```python
from build123d import *

# Parameters (mm, degrees)
SKETCH1_W           = 220
SKETCH1_H           = 30
BOSS_EXTRUDE1_DEPTH = 10
SKETCH2_W           = 23.523691572
SKETCH2_H           = 30
SKETCH2_R           = 11.1
BOSS_EXTRUDE3_DEPTH = 10
SKETCH6_R           = 1.5
CUT_EXTRUDE2_DEPTH  = 10
CUT_EXTRUDE3_START  = -10
SKETCH4_R           = 4
CUT_EXTRUDE3_DEPTH  = 4
SKETCH7_R           = 1.5
CUT_EXTRUDE4_DEPTH  = 14
CUT_EXTRUDE5_DEPTH  = 10
FILLET1_R           = 10


with BuildPart() as part:
    # Sketch1 → Boss-Extrude1 (new body)
    with BuildSketch(Plane(origin=(0, 0, 0), x_dir=(1, 0, 0), z_dir=(0, 1, 0))):
        Rectangle(SKETCH1_W, SKETCH1_H)
    extrude(amount=BOSS_EXTRUDE1_DEPTH)

    # Sketch2 → Boss-Extrude3 (add)
    with BuildSketch(Plane(origin=(0, 10, 0), x_dir=(1, 0, 0), z_dir=(0, 1, 0))):
        with Locations((-98.238154214, 0)):
            Rectangle(SKETCH2_W, SKETCH2_H)
        with Locations(Location((-98.238154214, 0, 0), (0, 0, 270))):
            Circle(SKETCH2_R, mode=Mode.SUBTRACT)
    extrude(amount=BOSS_EXTRUDE3_DEPTH)

    # Sketch6 → Cut-Extrude2 (cut)
    with BuildSketch(Plane.XY.offset(15)):
        with Locations((-98.238154214, 15)):
            Circle(SKETCH6_R)
    extrude(amount=-CUT_EXTRUDE2_DEPTH, mode=Mode.SUBTRACT)

    # Sketch4 → Cut-Extrude3 (cut)
    with BuildSketch(Plane(origin=(0, 10, 0), x_dir=(1, 0, 0), z_dir=(0, 1, 0)).offset(CUT_EXTRUDE3_START)):
        with Locations(Location((90, 0, 0), (0, 0, 90))):
            Circle(SKETCH4_R)
    extrude(amount=CUT_EXTRUDE3_DEPTH, mode=Mode.SUBTRACT)

    # Sketch7 → Cut-Extrude4 (cut)
    with BuildSketch(Plane(origin=(0, 4, 0), x_dir=(-1, 0, 0), z_dir=(0, -1, 0))):
        with Locations(Location((-90, 0, 0), (0, 0, 90))):
            Circle(SKETCH7_R)
    extrude(amount=-CUT_EXTRUDE4_DEPTH, mode=Mode.SUBTRACT)

    # Sketch8 → Cut-Extrude5 (cut)
    with BuildSketch(Plane(origin=(0, 10, 0), x_dir=(1, 0, 0), z_dir=(0, 1, 0))):
        Polygon((110, -15), (110, 0), (95, -15), align=None)
        Polygon((110, 15), (95, 15), (110, 0), align=None)
    extrude(amount=-CUT_EXTRUDE5_DEPTH, mode=Mode.SUBTRACT)

    # Fillet1
    fillet1_edges = [part.edges().sort_by_distance(p)[0] for p in [
        (110, 5, 0),
        (95, 5, 15),
        (95, 5, -15),
    ]]
    fillet(fillet1_edges, radius=FILLET1_R)


solid = part.part
```
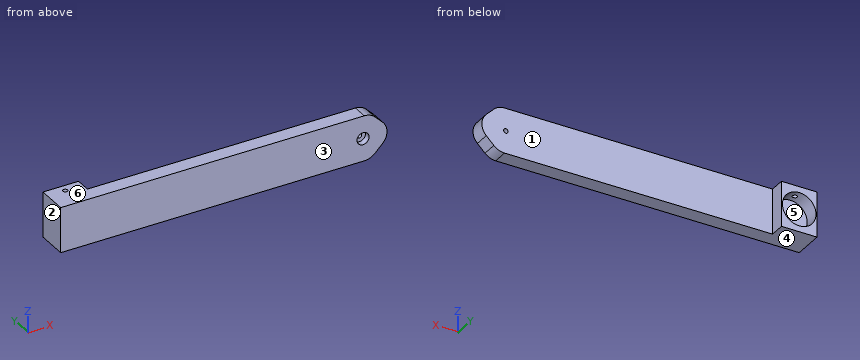
Geometry: final body of the model. Coordinates: model frame, mm. Face numbers are marked on the shaded views. A direction names the side the tool comes from. Coordinates: 2 decimals unless noted, no trailing zeros. Order: outer loops, then holes, each group sorted by start corner. A loop starts at its lowest first (then second) coordinate and runs counter-clockwise, first axis right, second up. Notation, with made-up numbers: M 42,46 L 86,46 A14 ccw 86,60 Z; hole C 88.25,-38.75 d10. An arc over 180 degrees is marked long. Answer in a Markdown table with one row per item. Add a question column.
Q1. Line query: L1, parallel to X at y = 14.75, z = 0; L2, parallel to Z at x = 90, y = 5.8; L3, parallel to Z at x = 90, y = 2. Output: solid intervals per line, ascending.
Q2. Section query A-A on x = 35.5. Return the cut outline in (y, z), and give its area (3 significant figures).
Q3. Mould query, pull axis Z, two halves, no side actions, for the marked faces 3, 4, 5 and 6. Classes: released by +Z, released by -Z, zero draft, split by the parting line, or undercut.
Q4. Contact query for flat-ended pins moving along their axis: P1, Ø1, axis at x = -11.5, z = -10, coming from the +Y side; P2, Ø3, axis at y = 17.5, z = 5, coming from the +X side; P3, Ø6.5, axis at x = 89, z = 1, coming from the -Y side; P4, Ø6.5, axis at x = 90, z = 0, coming from the -Y side. Output: stop coordinate, or through.
Q5. Reachability of the marked faces 1 and 2 from +Z, -Z, +X, -X, +Y, -Y: full face, straight path, thin tool, end or side. Return the list, or none.
Completed:
| question | item | result |
|---|---|---|
| 1 | L1 | x = -110 to -109.34, -87.14 to -86.48 |
| 1 | L2 | z = -15 to -1.5, 1.5 to 15 |
| 1 | L3 | z = -15 to -4, 4 to 15 |
| 2 | outline | M 0,-15 L 10,-15 L 10,15 L 0,15 Z |
| 2 | area | 300 mm2 |
| 3 | face 3 | zero draft |
| 3 | face 4 | released by -Z |
| 3 | face 5 | undercut |
| 3 | face 6 | released by +Z |
| 4 | P1 | stops at y = 10 |
| 4 | P2 | stops at x = -86.48 |
| 4 | P3 | stops at y = 0 |
| 4 | P4 | stops at y = 4 |
| 5 | face 1 | +Z, -Z, +X, +Y |
| 5 | face 2 | +Z, -Z, -X, +Y, -Y |
